Geometry: final body of the model. Coordinates: model frame, mm. Give positions to 0.01 mm unless a question says otherwise; leave off trailing zeros. Loops run counter-clockwise (first coordinate to the right, second up) from the corner with the lowest first, then second, coordinate; pieces in that order, holes last. Notation, with made-up numbers: (-23, -3.75) -> (-15, -3.75) arc R14 cw to (-15, 18.25) -> close; hole circle Ø6 at (52, -30.5). An arc over 180 degrees is marked (long way). Answer in a Markdown table with one row per item. Add a question column.
from build123d import *

# Parameters (mm, degrees)
SKETCH1_W           = 120.675
SKETCH1_H           = 1.5875
CUT_EXTRUDE2_START  = 19.25
SKETCH4_R           = 12.7
CUT_EXTRUDE2_DEPTH  = 22.225
BOSS_EXTRUDE1_START = -120.675
SKETCH5_R           = 7.9375
BOSS_EXTRUDE1_DEPTH = 120.675


with BuildPart() as part:
    # Sketch1 → Revolve1 (revolve)
    with BuildSketch(Plane(origin=(0, 0, 0), x_dir=(1, 0, 0), z_dir=(0, 1, 0))):
        with Locations((79.5875, 8.73125)):
            Rectangle(SKETCH1_W, SKETCH1_H)
    revolve(axis=Axis((157.324, 0, 0), (-1, 0, 0)))

    # Sketch4 → Cut-Extrude2 (cut)
    with BuildSketch(Plane(origin=(0, 0, 0), x_dir=(0, 0, -1), z_dir=(1, 0, 0)).offset(CUT_EXTRUDE2_START)):
        Circle(SKETCH4_R)
        Polygon((-9.235721046, 0.808020891), (-8.681700155, 0.254), (-8.681700155, -0.254), (-9.235721046, -0.808020891), (-8.593912259, -1.257420242), (-8.505698985, -1.75770258), (-8.955098336, -2.399511367), (-8.245002688, -2.730634406), (-8.071256455, -3.207998257), (-8.402379494, -3.918093905), (-7.645572882, -4.120879625), (-7.391572882, -4.56082053), (-7.594358603, -5.317627141), (-6.813836213, -5.385914002), (-6.487300108, -5.775064579), (-6.555586968, -6.555586968), (-5.775064579, -6.487300108), (-5.385914002, -6.813836213), (-5.317627141, -7.594358603), (-4.56082053, -7.391572882), (-4.120879625, -7.645572882), (-3.918093905, -8.402379494), (-3.207998257, -8.071256455), (-2.730634406, -8.245002688), (-2.399511367, -8.955098336), (-1.75770258, -8.505698985), (-1.257420242, -8.593912259), (-0.808020891, -9.235721046), (-0.254, -8.681700155), (0.254, -8.681700155), (0.808020891, -9.235721046), (1.257420242, -8.593912259), (1.75770258, -8.505698985), (2.399511367, -8.955098336), (2.730634406, -8.245002688), (3.207998257, -8.071256455), (3.918093905, -8.402379494), (4.120879625, -7.645572882), (4.56082053, -7.391572882), (5.317627141, -7.594358603), (5.385914002, -6.813836213), (5.775064579, -6.487300108), (6.555586968, -6.555586968), (6.487300108, -5.775064579), (6.813836213, -5.385914002), (7.594358603, -5.317627141), (7.391572882, -4.56082053), (7.645572882, -4.120879625), (8.402379494, -3.918093905), (8.071256455, -3.207998257), (8.245002688, -2.730634406), (8.955098336, -2.399511367), (8.505698985, -1.75770258), (8.593912259, -1.257420242), (9.235721046, -0.808020891), (8.681700155, -0.254), (8.681700155, 0.254), (9.235721046, 0.808020891), (8.593912259, 1.257420242), (8.505698985, 1.75770258), (8.955098336, 2.399511367), (8.245002688, 2.730634406), (8.071256455, 3.207998257), (8.402379494, 3.918093905), (7.645572882, 4.120879625), (7.391572882, 4.56082053), (7.594358603, 5.317627141), (6.813836213, 5.385914002), (6.487300108, 5.775064579), (6.555586968, 6.555586968), (5.775064579, 6.487300108), (5.385914002, 6.813836213), (5.317627141, 7.594358603), (4.56082053, 7.391572882), (4.120879625, 7.645572882), (3.918093905, 8.402379494), (3.207998257, 8.071256455), (2.730634406, 8.245002688), (2.399511367, 8.955098336), (1.75770258, 8.505698985), (1.257420242, 8.593912259), (0.808020891, 9.235721046), (0.254, 8.681700155), (-0.254, 8.681700155), (-0.808020891, 9.235721046), (-1.257420242, 8.593912259), (-1.75770258, 8.505698985), (-2.399511367, 8.955098336), (-2.730634406, 8.245002688), (-3.207998257, 8.071256455), (-3.918093905, 8.402379494), (-4.120879625, 7.645572882), (-4.56082053, 7.391572882), (-5.317627141, 7.594358603), (-5.385914002, 6.813836213), (-5.775064579, 6.487300108), (-6.555586968, 6.555586968), (-6.487300108, 5.775064579), (-6.813836213, 5.385914002), (-7.594358603, 5.317627141), (-7.391572882, 4.56082053), (-7.645572882, 4.120879625), (-8.402379494, 3.918093905), (-8.071256455, 3.207998257), (-8.245002688, 2.730634406), (-8.955098336, 2.399511367), (-8.505698985, 1.75770258), (-8.593912259, 1.257420242), align=None, mode=Mode.SUBTRACT)
    extrude(amount=CUT_EXTRUDE2_DEPTH, mode=Mode.SUBTRACT)

    # Sketch5 → Boss-Extrude1 (add)
    with BuildSketch(Plane(origin=(139.925, 0, 0), x_dir=(0, 0, -1), z_dir=(1, 0, 0)).offset(BOSS_EXTRUDE1_START)):
        Circle(SKETCH5_R)
    extrude(amount=BOSS_EXTRUDE1_DEPTH)


solid = part.part
(1) Cut plane A-A on x = 72. Return the cut outline in (y, z) (3 decimals), then the cut area to 3 significant figures.
(2) Material intervals for line 1 along Y through (x, z) = (95.5, 0.25); line 2 along X through (y, z) = (8.25, -3.5) (3 decimals); line 3 along Z through (x, y) = (129, -3.25), sorted ascending. Write a range as from..to.
(3) Pin query (flat end, axial travel): pin 1 Ø6 at (x, y) = (32.5, -7.5) entering from +Z; pin 2 Ø4 at (x, y) = (61, 5) entering from +Z; pin 3 Ø1.5 at (x, y) = (51.5, -4) entering from -Z; pin 4 Ø5 at (x, z) = (118.5, -0.5) entering from +Y (3 decimals). Return the tip coordinate at first contact, or that it passes through.
Answer list:
| question | item | result |
|---|---|---|
| 1 | outline | circle Ø19.05 at (0, 0) |
| 1 | area | 285 mm² |
| 2 | line 1 | y = -9.52..9.52 |
| 2 | line 2 | x = 41.475..139.925 |
| 2 | line 3 | z = -8.95..8.95 |
| 3 | pin 1 | stops at z = 7.59 |
| 3 | pin 2 | stops at z = 9.04 |
| 3 | pin 3 | stops at z = -8.95 |
| 3 | pin 4 | stops at y = 9.525 |
